from build123d import *

# Parameters (mm, degrees)
SKETCH1_R           = 3.375
BOSS_EXTRUDE1_DEPTH = 41.5
SKETCH2_R           = 2.5
BOSS_EXTRUDE2_DEPTH = 10.5
CUT_EXTRUDE1_START  = -5
SKETCH3_R           = 3.375
SKETCH3_R_2         = 1.5
CUT_EXTRUDE1_DEPTH  = 5


with BuildPart() as part:
    # Sketch1 → Boss-Extrude1 (new body)
    with BuildSketch(Plane(origin=(0, 0, 0), x_dir=(1, 0, 0), z_dir=(0, 1, 0))):
        with Locations(Location((0, 0, 0), (0, 0, 270))):
            Circle(SKETCH1_R)
    extrude(amount=BOSS_EXTRUDE1_DEPTH)

    # Sketch2 → Boss-Extrude2 (add)
    with BuildSketch(Plane(origin=(0, 41.5, 0), x_dir=(1, 0, 0), z_dir=(0, 1, 0))):
        with Locations(Location((0, 0, 0), (0, 0, 90))):
            Circle(SKETCH2_R)
    extrude(amount=BOSS_EXTRUDE2_DEPTH)

    # Sketch3 → Cut-Extrude1 (cut)
    with BuildSketch(Plane(origin=(0, 41.5, 0), x_dir=(1, 0, 0), z_dir=(0, 1, 0)).offset(CUT_EXTRUDE1_START)):
        with Locations(Location((0, 0, 0), (0, 0, 270))):
            Circle(SKETCH3_R)
        with Locations(Location((0, 0, 0), (0, 0, 270))):
            Circle(SKETCH3_R_2, mode=Mode.SUBTRACT)
    extrude(amount=CUT_EXTRUDE1_DEPTH, mode=Mode.SUBTRACT)


solid = part.part
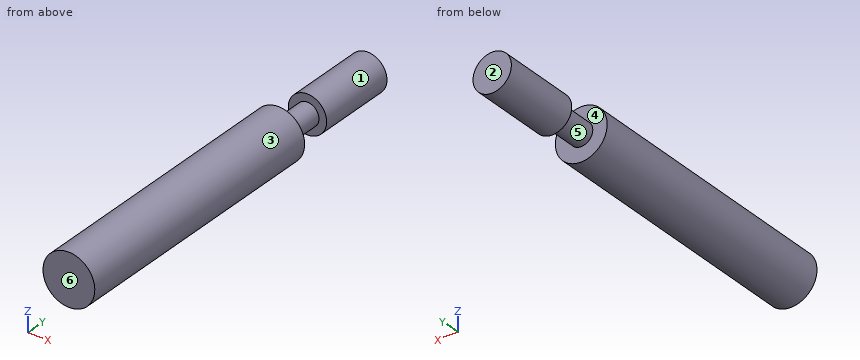
CAD build for the part. Positions are in the model's coordinates, mm. Face numbers are marked on the shaded views. A direction names the side the tool comes from. Round coordinates to 2 decimals unless told otherwise and drop trailing zeros. Order: outer loops, then holes, each group sorted by start corner. A loop starts at its lowest first (then second) coordinate and runs counter-clockwise, first axis right, second up. Notation, with made-up numbers: (-10, 50) - (34, 50) arc R30 cw to (34, 76) - close; hole circle Ø5 at (-3.5, 55.25). An arc over 180 degrees is marked (long way). Return JSON: item names as keys, results as strings.
(1) Pull direction Y, two halves, no side cores. Call the marked faces 3, 4, 5 and 6: +Y half, -Y half, draft (parallel to the pull), parting line (faces both ways), or undercut.
Answer key:
{"face 3": "draft", "face 4": "undercut", "face 5": "undercut", "face 6": "-Y half"}
(2) Cut at C-C (z = -2). Give the cut face in (x, y), then the cut area to 3 significant figures.
Answer key:
{"outline": "(-2.72, 0) - (2.72, 0) - (2.72, 36.5) - (-2.72, 36.5) - close; (-1.5, 41.5) - (1.5, 41.5) - (1.5, 52) - (-1.5, 52) - close", "area": "230 mm^2"}
(3) Wall check: probe 1 along Y at (x, z) = (-1, -1.25); probe 2 along Y at (x, z) = (2.5, 0.75); probe 3 along X at (y, z) = (27.5, -0.25). Give the ranges that are in metal, low to high. Write a range as from..to.
Answer key:
{"probe 1": "y = 0..36.5, 41.5..52", "probe 2": "y = 0..36.5", "probe 3": "x = -3.37..3.37"}
(4) Cut at D-D (y = 37). Give the cut face in (x, z), then the cut area to 3 significant figures.
Answer key:
{"outline": "circle Ø3 at (0, 0)", "area": "7.07 mm^2"}
(5) Pin check, flat tips, straight feed: pin 1 Ø3 at (x, y) = (-2.5, 9) entering from -Z; pin 2 Ø1.5 at (y, z) = (23.5, 2.5) entering from +X; pin 3 Ø1 at (y, z) = (12, -2) entering from -X. Stop position of each tip, or through.
Answer key:
{"pin 1": "stops at z = -3.22", "pin 2": "stops at x = 2.89", "pin 3": "stops at x = -3.02"}
(6) Cut at B-B (x = 0). Give the cut face in (y, z) (3 decimals), then the cut area to 3 significant figures.
Answer key:
{"outline": "(0, -3.375) - (36.5, -3.375) - (36.5, -1.5) - (41.5, -1.5) - (41.5, -2.5) - (52, -2.5) - (52, 2.5) - (41.5, 2.5) - (41.5, 1.5) - (36.5, 1.5) - (36.5, 3.375) - (0, 3.375) - close", "area": "314 mm^2"}
(7) Tool access for the marked faces 1 and 2: list every direction of +Z, -Z, +X, -X, +Y, -Y with a clear straight run to the whole face (end or side of a thin tool).
Answer key:
{"face 1": "+Y", "face 2": "+Z, -Z, +X, -X, +Y"}
(8) Cut at A-A (z = 0). Give the cut face in (x, y) (3 decimals).
Answer key:
{"outline": "(-3.375, 0) - (3.375, 0) - (3.375, 36.5) - (1.5, 36.5) - (1.5, 41.5) - (2.5, 41.5) - (2.5, 52) - (-2.5, 52) - (-2.5, 41.5) - (-1.5, 41.5) - (-1.5, 36.5) - (-3.375, 36.5) - close"}
